Build history of the part. All positions in model axes, mm. A direction names the side the tool comes from. Give positions to 0.01 mm unless a question says otherwise; leave off trailing zeros. Write each loop counter-clockwise with the first axis right and the second up, starting at its lowest first coordinate (ties: lowest second). Pieces come first, ordered by that corner, then holes.
from build123d import *

# Parameters (mm, degrees)
F1_DEPTH = 63.5
F2_DEPTH = 25.4
F3_DEPTH = 7.9375


with BuildPart() as f1:
    # F0 (on Front) → F1 (new body, symmetric)
    with BuildSketch(Plane.XZ):
        Polygon((-41.275, 9.525), (-41.275, -9.525), (41.275, -9.525), (41.275, 9.525), (22.225, 9.525), align=None)
    extrude(amount=F1_DEPTH, both=True)

    # F0 (on Front) → F2 (join, symmetric)
    with BuildSketch(Plane.XZ):
        with BuildLine():
            Line((22.225, 9.525), (41.275, 9.525))
            Line((41.275, 9.525), (41.275, 27.0002))
            ThreePointArc((41.275, 27.0002), (45.92468, 38.22552), (57.15, 42.8752))
            Line((57.15, 42.8752), (72.076506, 42.8752))
            Line((72.076506, 42.8752), (72.076506, 61.9252))
            Line((72.076506, 61.9252), (57.15, 61.9252))
            ThreePointArc((57.15, 61.9252), (32.454296, 51.695904), (22.225, 27.0002))
            Line((22.225, 27.0002), (22.225, 9.525))
        make_face()
    extrude(amount=F2_DEPTH, both=True)

    # F0 (on Front) → F3 (join, symmetric)
    with BuildSketch(Plane.XZ):
        with BuildLine():
            add(Edge.make_bspline(
                [(-41.275, 9.525), (-38.149111, 39.227815), (15.005312, 62.741945), (57.15, 61.9252)],
                knots=[0, 0, 0, 0, 111.504536, 111.504536, 111.504536, 111.504536], degree=3))
            Line((-41.275, 9.525), (22.225, 9.525))
            Line((22.225, 9.525), (22.225, 27.0002))
            ThreePointArc((22.225, 27.0002), (32.454296, 51.695904), (57.15, 61.9252))
        make_face()
    extrude(amount=F3_DEPTH, both=True)

    # F0 (on Front) → F4 (revolve)
    with BuildSketch(Plane.XZ):
        Polygon((105.234338, 66.675), (105.234338, 61.9252), (105.234338, 42.8752), (105.234338, 38.1), (122.876506, 38.1), (122.876506, 66.675), align=None)
    revolve(axis=Axis((72.076506, 0, 52.3875), (0, 0, 1)))


solid = f1.part
1. Mould opens along X. For faces 6 (the face through (44, -7.938, 60)), 7 (the face through (31, -25.4, 24)), 8 (the face through (41.275, -1, 4)) say: pulls with the +X half, pulls with the -X half, needs draft (parallel to the pull), parting line crosses it, or undercut.
2. Drill centre lines: line 1 along X through (y, z) = (-54, -4.5) (3 decimals); line 2 along Z through (x, y) = (8, 28) (3 decimals); line 3 along Y through (x, z) = (20.5, 10). Where is each one in solid material? Low to high.
3. Saw through at A-A on y = -41. Give the cut face in (x, z) (1 decimal).
4. Saw through at B-B on x = 74.5. Give the cut face in (y, z) (3 decimals), plus the area to 3 significant figures.
5. 3-axis set-ups, long thin cutter, end or side, ignore diameter. For faces 1 (the face through (-1, 63.5, 0)), 2 (the face through (72.077, 0, 52)), 3 (the face through (65, 0, 42.875)), 4 (the face through (65, 0, 61.925)), 5 (the face through (83, -33, 66.675)): which of +Z, -Z, +X, -X, +Y, -Y reach the whole face in a straight line?
6. Saw through at C-C on z = 5. Give the cut face in (x, y) (3 decimals), plus the area to 3 significant figures.
7. Drop flat-ended pins along their axis: pin 1 (10 mm diameter, centred on x = 60, z = 54.5, fed in from +Y); pin 2 (3 mm diameter, centred on x = 94, y = 46, fed in from -Z); pin 3 (12 mm diameter, centred on x = 38.5, z = 36, fed in from -Y); pin 4 (9.5 mm diameter, centred on y = -4, z = 50, fed in from +X). Give the stop position or say it passes through.
Outcome:
1. face 6: undercut
1. face 7: needs draft
1. face 8: pulls with the +X half
2. line 1: x = -41.275 to 41.275
2. line 2: z = -9.525 to 9.525
2. line 3: y = -7.94 to 7.94
3. outline: (-41.3, -9.5) - (41.3, -9.5) - (41.3, 9.5) - (-41.3, 9.5) - close; (42.1, 38.1) - (102.1, 38.1) - (102.1, 66.7) - (42.1, 66.7) - close
4. outline: (-50.742, 38.1) - (-33.069, 38.1) - (-33.069, 66.675) - (-50.742, 66.675) - close; (33.069, 38.1) - (50.742, 38.1) - (50.742, 66.675) - (33.069, 66.675) - close
4. area: 1,010 mm2
5. face 1: +Z, -Z, +X, -X, +Y
5. face 2: +Z, -Z
5. face 3: -Z
5. face 4: +Z
5. face 5: +Z, +X, -X, +Y, -Y
6. outline: (-41.275, -63.5) - (41.275, -63.5) - (41.275, 63.5) - (-41.275, 63.5) - close
6. area: 10,500 mm2
7. pin 1: stops at y = 50.3
7. pin 2: stops at z = 38.1
7. pin 3: stops at y = -42.42
7. pin 4: stops at x = 122.88
